```python
from build123d import *

# Parameters (mm, degrees)
SKETCH_2_R           = 0.825
SKETCH_2_R_2         = 6
EXTRUDE_1_DEPTH      = 2
SKETCH_4_R           = 1.6
CUT_EXTRUDE_1_DEPTH  = 15
EXTRUDE_2_DEPTH      = 2
EXTRUDE_3_DEPTH      = 2
SKETCH_21_W          = 94.174920184
SKETCH_21_H          = 20
EXTRUDE_5_DEPTH      = 4
CUT_EXTRUDE_10_DEPTH = 7
SKETCH_23_W          = 30
SKETCH_23_H          = 8.450093073
CUT_EXTRUDE_11_DEPTH = 7
CHAMFER_START        = -2
CHAMFER_6_DEPTH      = 4
SKETCH_25_R          = 1.6
CUT_EXTRUDE_12_DEPTH = 7
FILLET_3_R           = 3
CUT_EXTRUDE_13_DEPTH = 32
SKETCH_27_R          = 1.621448002
CUT_EXTRUDE_14_DEPTH = 32


with BuildPart() as part:
    # 草图2 → 凸台-拉伸1 (new, symmetric)
    with BuildSketch(Plane.XY):
        Polygon((10.355339059, 25), (-10.355339059, 25), (-25, 10.355339059), (-25, -10.355339059), (-10.355339059, -25), (10.355339059, -25), (25, -10.355339059), (25, 10.355339059), align=None)
        with Locations((-16.5, 0)):
            Circle(SKETCH_2_R, mode=Mode.SUBTRACT)
        with Locations((0, 16.5)):
            Circle(SKETCH_2_R, mode=Mode.SUBTRACT)
        with Locations((16.5, 0)):
            Circle(SKETCH_2_R, mode=Mode.SUBTRACT)
        with Locations((0, -16.5)):
            Circle(SKETCH_2_R, mode=Mode.SUBTRACT)
        Circle(SKETCH_2_R_2, mode=Mode.SUBTRACT)
    extrude(amount=EXTRUDE_1_DEPTH, both=True)

    # 草图4 → 切除-拉伸1 (cut)
    with BuildSketch(Plane(origin=(0, 0, -2), x_dir=(-1, 0, 0), z_dir=(0, 0, -1))):
        with Locations((-7.5, -20)):
            Circle(SKETCH_4_R)
        with Locations(Location((7.5, -20, 0), (0, 0, 180))):
            Circle(SKETCH_4_R)
        with Locations((-20, 7.5)):
            Circle(SKETCH_4_R)
        with Locations(Location((-20, -7.5, 0), (0, 0, 180))):
            Circle(SKETCH_4_R)
        with Locations((7.5, 20)):
            Circle(SKETCH_4_R)
        with Locations(Location((-7.5, 20, 0), (0, 0, 180))):
            Circle(SKETCH_4_R)
        with Locations((20, -7.5)):
            Circle(SKETCH_4_R)
        with Locations(Location((20, 7.5, 0), (0, 0, 180))):
            Circle(SKETCH_4_R)
    extrude(amount=-CUT_EXTRUDE_1_DEPTH, mode=Mode.SUBTRACT)

    # 草图5 → 凸台-拉伸2 (add, symmetric)
    with BuildSketch(Plane.XY):
        Polygon((-25, -10.355339059), (-80, -73), (-60, -73), (-11.17766953, -24.17766953), align=None)
        Polygon((60, -73), (80, -73), (25, -10.355339059), (11.17766953, -24.17766953), align=None)
    extrude(amount=EXTRUDE_2_DEPTH, both=True)

    # 草图6 → 凸台-拉伸3 (add, symmetric)
    with BuildSketch(Plane.XY):
        Polygon((-60, -73), (-35, -73), (-10.355339059, -25), (-11.17766953, -24.17766953), align=None)
        Polygon((60, -73), (11.17766953, -24.17766953), (10.355339059, -25), (35, -73), align=None)
    extrude(amount=EXTRUDE_3_DEPTH, both=True)

    # 草图21 → 凸台-拉伸5 (add)
    with BuildSketch(Plane.XY.offset(2)):
        with Locations((0, -63)):
            Rectangle(SKETCH_21_W, SKETCH_21_H)
    extrude(amount=-EXTRUDE_5_DEPTH)

    # 草图22 → 切除-拉伸10 (cut, symmetric)
    with BuildSketch(Plane.XY.offset(2)):
        with BuildLine():
            Line((-72.098289103, -64), (-93.602322684, -86.771790357))
            Line((-93.602322684, -86.771790357), (107.138572214, -85.642128596))
            Line((107.138572214, -85.642128596), (72.098289103, -64))
            add(Edge.make_bspline(
                [(-72.098289103, -64), (0, -76), (72.098289103, -64)],
                knots=[0, 0, 0, 1, 1, 1], degree=2))
        make_face()
    extrude(amount=CUT_EXTRUDE_10_DEPTH, both=True, mode=Mode.SUBTRACT)

    # 草图23 → 切除-拉伸11 (cut, symmetric)
    with BuildSketch(Plane.XY.offset(2)):
        with Locations((0, -69.225046537)):
            Rectangle(SKETCH_23_W, SKETCH_23_H)
    extrude(amount=CUT_EXTRUDE_11_DEPTH, both=True, mode=Mode.SUBTRACT)

    # 倒角6: read off the stored shape, not the designer's step
    # 倒角6 outline → 倒角6 (cut)
    with BuildSketch(Plane.XY.offset(CHAMFER_START)):
        with BuildLine():
            Line((72.098289103, -64), (62.861553298, -53.47941486))
            Line((62.861553298, -53.47941486), (23.982189464, -69.336136194))
            add(Edge.make_bspline(
                [(72.098289103, -64), (48.040239283, -68.004208719), (23.982189464, -69.336136194)],
                knots=[0, 0, 0, 0.33368406, 0.33368406, 0.33368406], degree=2))
        make_face()
        with BuildLine():
            Line((-23.982189464, -69.336136194), (-62.861553298, -53.47941486))
            Line((-62.861553298, -53.47941486), (-72.098289103, -64))
            add(Edge.make_bspline(
                [(-23.982189464, -69.336136194), (-48.040239283, -68.004208719), (-72.098289103, -64)],
                knots=[0.66631594, 0.66631594, 0.66631594, 1, 1, 1], degree=2))
        make_face()
    extrude(amount=CHAMFER_6_DEPTH, mode=Mode.SUBTRACT)

    # 草图25 → 切除-拉伸12 (cut, symmetric)
    with BuildSketch(Plane.XY.offset(2)):
        with Locations((-52.235249282, -53.148500686)):
            Circle(SKETCH_25_R)
        with Locations((-38.268733006, -58.619919434)):
            Circle(SKETCH_25_R)
        with Locations((38.268733006, -58.619919434)):
            Circle(SKETCH_25_R)
        with Locations((52.235249282, -53.148500686)):
            Circle(SKETCH_25_R)
    extrude(amount=CUT_EXTRUDE_12_DEPTH, both=True, mode=Mode.SUBTRACT)

    # 圆角3
    fillet_3_edges = [part.edges().sort_by_distance(p)[0] for p in [
        (-15, -69.740292883, -3e-07),
        (15, -69.740292883, -3e-07),
    ]]
    fillet(fillet_3_edges, radius=FILLET_3_R)

    # 草图26 → 切除-拉伸13 (cut, symmetric)
    with BuildSketch(Plane(origin=(0, 0, 0), x_dir=(0, 0, -1), z_dir=(1, 0, 0))):
        with BuildLine():
            Line((-2, -69.366736418), (-2.263749967, -70.210945681))
            Line((-2.263749967, -70.210945681), (2.547301332, -70.18897741))
            Line((2.547301332, -70.18897741), (2, -69.366736418))
            add(Edge.make_bspline(
                [(-2, -69.366736418), (0, -69.686845507), (2, -69.366736418)],
                knots=[0, 0, 0, 1, 1, 1], degree=2))
        make_face()
    extrude(amount=CUT_EXTRUDE_13_DEPTH, both=True, mode=Mode.SUBTRACT)

    # 草图27 → 切除-拉伸14 (cut, symmetric)
    with BuildSketch(Plane(origin=(0, 0, -2), x_dir=(-1, 0, 0), z_dir=(0, 0, -1))):
        with Locations(Location((-7.5, -59.5, 0), (0, 0, 180))):
            Circle(SKETCH_27_R)
        with Locations(Location((7.5, -59.5, 0), (0, 0, 180))):
            Circle(SKETCH_27_R)
    extrude(amount=CUT_EXTRUDE_14_DEPTH, both=True, mode=Mode.SUBTRACT)


solid = part.part
```
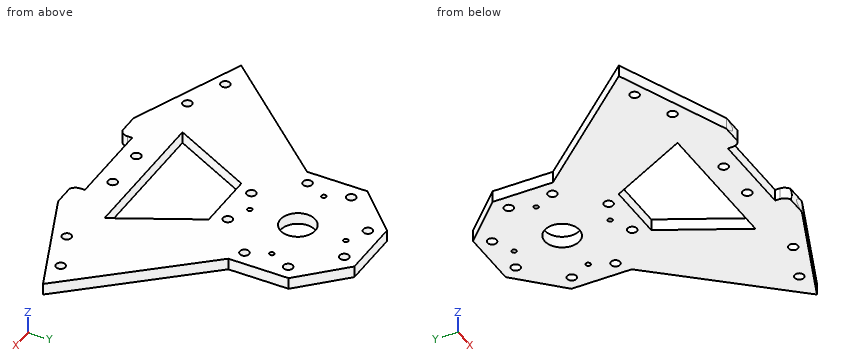
Work out the finished part from the listing and answer in its coordinate system (mm). Coordinates: 2 decimals unless noted, no trailing zeros. Order: outer loops, then holes, each group sorted by start corner. A loop starts at its lowest first (then second) coordinate and runs counter-clockwise, first axis right, second up. Notation, with made-up numbers: (-4.75, 70.5) - (32.25, 70.5) arc R20 cw to (32.25, 109.5) - close; hole circle Ø10 at (-16, 47). An arc over 180 degrees is marked (long way). Answer as a JSON object with one key per item and string values.
1. Find section A-A on y = 7.5. Determine the outline of the cut face in (x, z).
Output values:
{"outline": "(-25, -2) - (-21.6, -2) - (-21.6, 2) - (-25, 2) - close; (-18.4, -2) - (18.4, -2) - (18.4, 2) - (-18.4, 2) - close; (21.6, -2) - (25, -2) - (25, 2) - (21.6, 2) - close"}
2. Consider line 1 (Y direction, x = 7.5, z = 0); line 2 (X direction, y = 1, z = 1.2); line 3 (Y direction, x = -8, z = 0.3). Determine where each line is inside the solid, lowest interval first.
Output values:
{"line 1": "y = -65 to -61.12, -57.88 to -53, -25 to -21.6, -18.4 to 18.4, 21.6 to 25", "line 2": "x = -25 to -5.92, 5.92 to 25", "line 3": "y = -65 to -61.04, -57.96 to -53, -25 to -21.52, -18.48 to 18.48, 21.52 to 25"}
3. Each of these flat-tipped pins is pushed along its axis until it touches: P1, Ø1.2, axis at x = -5, z = 0, coming from the -Y side; P2, Ø1.3, axis at y = -66, z = 0, coming from the -X side; P3, Ø1, axis at x = 0, y = 16.5, coming from the +Z side; P4, Ø1.3, axis at y = -66, z = 1, coming from the +X side. Where does it stop, or does it pass through?
Output values:
{"P1": "stops at y = -65", "P2": "stops at x = -33.76", "P3": "passes through", "P4": "stops at x = 33.76"}
4. Find section B-B on x = -7.5. Determine the outline of the cut face in (y, z), plus the area to 3 significant figures.
Output values:
{"outline": "(-65, -2) - (-61.12, -2) - (-61.12, 2) - (-65, 2) - close; (-57.88, -2) - (-53, -2) - (-53, 2) - (-57.88, 2) - close; (-25, -2) - (-21.6, -2) - (-21.6, 2) - (-25, 2) - close; (-18.4, -2) - (18.4, -2) - (18.4, 2) - (-18.4, 2) - close; (21.6, -2) - (25, -2) - (25, 2) - (21.6, 2) - close", "area": "209 mm²"}
5. Find section D-D on z = -1.35. Count the separate pieces of the cut face and the enclosed holes in it, plus the area to 3 significant figures.
Output values:
{"separate pieces": "1", "enclosed holes": "20", "area": "5,370 mm²"}
6. Find section C-C on y = -45.5. Determine the outline of the cut face in (x, z), plus the area to 3 significant figures.
Output values:
{"outline": "(-55.86, -2) - (-20.88, -2) - (-20.88, 2) - (-55.86, 2) - close; (20.88, -2) - (55.86, -2) - (55.86, 2) - (20.88, 2) - close", "area": "280 mm²"}
